Here's how the part is built. I have some questions about the finished solid (model axes, mm). Face numbers are marked on the shaded views. Round coordinates to 2 decimals unless told otherwise and drop trailing zeros. Order: outer loops, then holes, each group sorted by start corner. A loop starts at its lowest first (then second) coordinate and runs counter-clockwise, first axis right, second up. Notation, with made-up numbers: M 79,61.25 L 104,61.25 A13 ccw 104,65.25 Z; hole C 70.5,62.5 d1. An arc over 180 degrees is marked long. Write item = value, one per line. Start each with the question number.
Item 1: Please list where these lines run through material, in increasing order: L1, parallel to Y at x = 0, z = 1.55; L2, parallel to Y at x = 0, z = -0.5; L3, parallel to Z at x = -9, y = -10.5.
Item 2: I'm going to push a flat-ended pin straight in: P1, Ø2, axis at x = -1, z = 1.5, coming from the -Y side. Where does the tip first touch, or does it pass through?
Item 3: I want a section at C-C, the plane z = 2.05. List the corners of the cut face in (x, y) for me.
Item 4: We'd pull the mould along Y, two halves only. Please class the marked faces 1, 2 and 3: pulls with the +Y half, pulls with the -Y half, needs draft (parallel to the pull), parting line crosses it, or undercut.
Item 5: I want a section at A-A, the plane y = 0. List the corners of the cut face in (x, z) for me, plus the area to 3 significant figures.
Item 6: I want a section at D-D, the plane z = -1.5. List the corners of the cut face in (x, y) for me, plus the area to 3 significant figures.
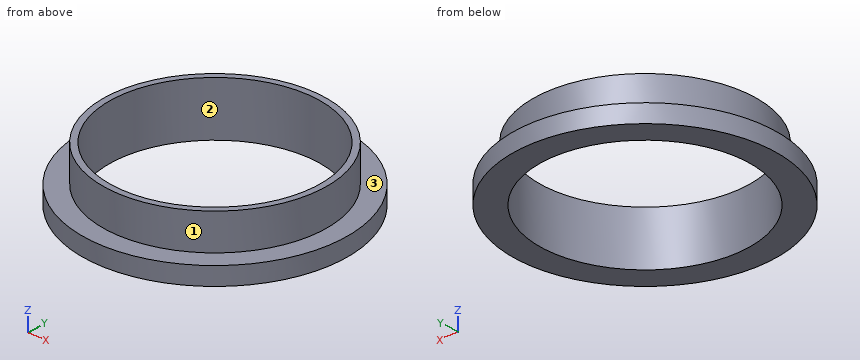
```python
from build123d import *

# Parameters (mm, degrees)
CROQUIS1_R              = 12.25
SALIENTE_EXTRUIR1_DEPTH = 4
CROQUIS2_R              = 14.5
SALIENTE_EXTRUIR2_DEPTH = 2
CROQUIS3_R              = 11.55
CORTAR_EXTRUIR1_DEPTH   = 10


with BuildPart() as part:
    # Croquis1 → Saliente-Extruir1 (new body)
    with BuildSketch(Plane.XY):
        Circle(CROQUIS1_R)
    extrude(amount=SALIENTE_EXTRUIR1_DEPTH)

    # Croquis2 → Saliente-Extruir2 (add)
    with BuildSketch(Plane(origin=(0, 0, 0), x_dir=(-1, 0, 0), z_dir=(0, 0, -1))):
        Circle(CROQUIS2_R)
    extrude(amount=SALIENTE_EXTRUIR2_DEPTH)

    # Croquis3 → Cortar-Extruir1 (cut)
    with BuildSketch(Plane(origin=(0, 0, -2), x_dir=(-1, 0, 0), z_dir=(0, 0, -1))):
        Circle(CROQUIS3_R)
    extrude(amount=-CORTAR_EXTRUIR1_DEPTH, mode=Mode.SUBTRACT)


solid = part.part
```
Filled in:
q1.L1 = -12.25 to -11.55, 11.55 to 12.25
q1.L2 = -14.5 to -11.55, 11.55 to 14.5
q1.L3 = -2 to 0
q2.P1 = -12.25
q3.outline = C 0,0 d24.5; hole C 0,0 d23.1
q4.face_1 = parting line crosses it
q4.face_2 = undercut
q4.face_3 = needs draft
q5.outline = M -14.5,-2 L -11.55,-2 L -11.55,4 L -12.25,4 L -12.25,0 L -14.5,0 Z; M 11.55,-2 L 14.5,-2 L 14.5,0 L 12.25,0 L 12.25,4 L 11.55,4 Z
q5.area = 17.4 mm^2
q6.outline = C 0,0 d29; hole C 0,0 d23.1
q6.area = 241 mm^2
